```python
from build123d import *

# Parameters (mm, degrees)
SKETCH1_W           = 125
SKETCH1_H           = 70
BOSS_EXTRUDE1_DEPTH = 5
FILLET1_R           = 1
CUT_EXTRUDE1_REACH  = 145.353
SKETCH2_R           = 1.5


with BuildPart() as part:
    # Sketch1 → Boss-Extrude1 (new body)
    with BuildSketch(Plane(origin=(0, 0, 0), x_dir=(1, 0, 0), z_dir=(0, 1, 0))):
        with Locations((62.5, 35)):
            Rectangle(SKETCH1_W, SKETCH1_H)
    extrude(amount=BOSS_EXTRUDE1_DEPTH)

    # Fillet1
    fillet1_edges = [part.edges().sort_by_distance(p)[0] for p in [
        (125, 5, -35),
        (62.5, 5, -70),
        (0, 5, -35),
        (62.5, 5, 0),
    ]]
    fillet(fillet1_edges, radius=FILLET1_R)

    # Sketch2 → Cut-Extrude1 (cut, up to next)
    with BuildSketch(Plane(origin=(0, 5, 0), x_dir=(1, 0, 0), z_dir=(0, 1, 0)), mode=Mode.PRIVATE) as cut_extrude1_sk1:
        with Locations(Location((120, 5, 0), (0, 0, 270))):
            Circle(SKETCH2_R)
    cut_extrude1_tool1 = extrude(cut_extrude1_sk1.sketch, amount=-CUT_EXTRUDE1_REACH, mode=Mode.PRIVATE) & part.part
    # Sketch2 → Cut-Extrude1 (cut, up to next)
    with BuildSketch(Plane(origin=(0, 5, 0), x_dir=(1, 0, 0), z_dir=(0, 1, 0)), mode=Mode.PRIVATE) as cut_extrude1_sk2:
        with Locations(Location((120, 65, 0), (0, 0, 90))):
            Circle(SKETCH2_R)
    cut_extrude1_tool2 = extrude(cut_extrude1_sk2.sketch, amount=-CUT_EXTRUDE1_REACH, mode=Mode.PRIVATE) & part.part
    # Sketch2 → Cut-Extrude1 (cut, up to next)
    with BuildSketch(Plane(origin=(0, 5, 0), x_dir=(1, 0, 0), z_dir=(0, 1, 0)), mode=Mode.PRIVATE) as cut_extrude1_sk3:
        with Locations(Location((5, 65, 0), (0, 0, 270))):
            Circle(SKETCH2_R)
    cut_extrude1_tool3 = extrude(cut_extrude1_sk3.sketch, amount=-CUT_EXTRUDE1_REACH, mode=Mode.PRIVATE) & part.part
    # Sketch2 → Cut-Extrude1 (cut, up to next)
    with BuildSketch(Plane(origin=(0, 5, 0), x_dir=(1, 0, 0), z_dir=(0, 1, 0)), mode=Mode.PRIVATE) as cut_extrude1_sk4:
        with Locations(Location((5, 5, 0), (0, 0, 90))):
            Circle(SKETCH2_R)
    cut_extrude1_tool4 = extrude(cut_extrude1_sk4.sketch, amount=-CUT_EXTRUDE1_REACH, mode=Mode.PRIVATE) & part.part
    add(cut_extrude1_tool1.solids().sort_by_distance((120, 5, -5))[0], mode=Mode.SUBTRACT)
    add(cut_extrude1_tool2.solids().sort_by_distance((120, 5, -65))[0], mode=Mode.SUBTRACT)
    add(cut_extrude1_tool3.solids().sort_by_distance((5, 5, -65))[0], mode=Mode.SUBTRACT)
    add(cut_extrude1_tool4.solids().sort_by_distance((5, 5, -5))[0], mode=Mode.SUBTRACT)


solid = part.part
```
Work out the finished part from the listing and answer in its coordinate system (mm). Give positions to 0.01 mm unless a question says otherwise; leave off trailing zeros. Write each loop counter-clockwise with the first axis right and the second up, starting at its lowest first coordinate (ties: lowest second). Pieces come first, ordered by that corner, then holes.
(1) Straight lines are drawn through the part: line 1 (Z direction, x = 120, y = 3.75); line 2 (X direction, y = 1.9, z = -5); line 3 (X direction, y = 4.65, z = -24). For each, find the intervals that lie inside material, in ascending order.
Final values:
line 1: z = -70 to -66.5, -63.5 to -6.5, -3.5 to 0
line 2: x = 0 to 3.5, 6.5 to 118.5, 121.5 to 125
line 3: x = 0.24 to 124.76
(2) A flat-ended cylindrical pin translates along its axis: pin 1 Ø2.5 at (x, z) = (5, -65) entering from +Y. Find the tip coordinate at first contact, or state that the pin passes through.
Final values:
pin 1: passes through
(3) The part is cut by section B-B on x = 120. Write down the section's boundary in (y, z).
Final values:
outline: (0, -70) - (4, -70) arc R1 ccw to (5, -69) - (5, -66.5) - (0, -66.5) - close; (0, -63.5) - (5, -63.5) - (5, -6.5) - (0, -6.5) - close; (0, -3.5) - (5, -3.5) - (5, -1) arc R1 ccw to (4, 0) - (0, 0) - close
(4) The part is cut by section A-A on z = -65. Write down the section's boundary in (x, y).
Final values:
outline: (0, 0) - (3.5, 0) - (3.5, 5) - (1, 5) arc R1 ccw to (0, 4) - close; (6.5, 0) - (118.5, 0) - (118.5, 5) - (6.5, 5) - close; (121.5, 0) - (125, 0) - (125, 4) arc R1 ccw to (124, 5) - (121.5, 5) - close
(5) The mould has two halves that part along Z. Classify faces 1 (the flat face through (62, 5, -35)), 2 (the flat face through (62, 2, 0)), 3 (the cylindrical face through (121.487, 2.535, -5.195)): pulls with the +Z half, pulls with the -Z half, needs draft (parallel to the pull), parting line crosses it, or undercut.
Final values:
face 1: needs draft
face 2: pulls with the +Z half
face 3: undercut
